from build123d import *

# Parameters (mm, degrees)
SKETCH_1_W          = 140
SKETCH_1_H          = 50
EXTRUDE_1_DEPTH     = 6
SKETCH_6_R          = 2.75
CUT_EXTRUDE_4_DEPTH = 7
SKETCH_5_W          = 140
SKETCH_5_H          = 12
EXTRUDE_3_DEPTH     = 2
M6X1_01_AT_2_COUNT  = 2
M6X1_01_AT_2_PITCH  = 50
M6X1_01_AT_3_COUNT  = 2
M6X1_01_AT_3_PITCH  = 50
SKETCH_4_W          = 9
SKETCH_4_H          = 26
CUT_EXTRUDE_2_DEPTH = 9


with BuildPart() as part:
    # Эскиз1 → Вытянуть1 (new body)
    with BuildSketch(Plane.XY):
        Rectangle(SKETCH_1_W, SKETCH_1_H)
    extrude(amount=EXTRUDE_1_DEPTH)

    # Эскиз6 → Вытянуть4 (cut, through all)
    with BuildSketch(Plane(origin=(0, 0, 0), x_dir=(-1, 0, 0), z_dir=(0, 0, -1))):
        with Locations((42, 19)):
            Circle(SKETCH_6_R)
        with Locations((14, 19)):
            Circle(SKETCH_6_R)
        with Locations((-14, 19)):
            Circle(SKETCH_6_R)
        with Locations((-42, 19)):
            Circle(SKETCH_6_R)
    extrude(amount=-CUT_EXTRUDE_4_DEPTH, mode=Mode.SUBTRACT)

    # Эскиз5 → Вытянуть3 (add)
    with BuildSketch(Plane(origin=(0, 0, 0), x_dir=(-1, 0, 0), z_dir=(0, 0, -1))):
        with Locations((0, -19)):
            Rectangle(SKETCH_5_W, SKETCH_5_H)
    extrude(amount=EXTRUDE_3_DEPTH)

    # Эскиз2 → Отверстие обработанное метчиком M6x1.01 (revolve, cut)
    with BuildSketch(Plane(origin=(0, -19, 6), x_dir=(0, -1, 0), z_dir=(1, 0, 0))):
        Polygon((0, 0), (0, 8.000025), (3.25, 8.000025), (2.5, 7.250025), (2.5, 0), align=None)
    m6x1_01 = revolve(axis=Axis((0, -19, 12.35), (0, 0, -1)), mode=Mode.SUBTRACT)

    # Отверстие обработанное метчиком M6x1.01 at 2: Отверстие обработанное метчиком M6x1.01 ×2
    with Locations(*[(-i * M6X1_01_AT_2_PITCH, 0, 0) for i in range(1, M6X1_01_AT_2_COUNT)]):
        add(m6x1_01, mode=Mode.SUBTRACT)

    # Отверстие обработанное метчиком M6x1.01 at 3: Отверстие обработанное метчиком M6x1.01 ×2
    with Locations(*[(i * M6X1_01_AT_3_PITCH, 0, 0) for i in range(1, M6X1_01_AT_3_COUNT)]):
        add(m6x1_01, mode=Mode.SUBTRACT)

    # Эскиз4 → Вытянуть2 (cut, through all)
    with BuildSketch(Plane.XY.offset(6)):
        with Locations((-65.5, 12)):
            Rectangle(SKETCH_4_W, SKETCH_4_H)
        with Locations((65.5, 12)):
            Rectangle(SKETCH_4_W, SKETCH_4_H)
    extrude(amount=-CUT_EXTRUDE_2_DEPTH, mode=Mode.SUBTRACT)


solid = part.part
Source: CAD feature listing. Evaluate the final solid. Frame: model axes, mm. A direction names the side the tool comes from. Coordinates: 2 decimals unless noted, no trailing zeros. Loops run counter-clockwise (first coordinate to the right, second up) from the corner with the lowest first, then second, coordinate; pieces in that order, holes last. Notation, with made-up numbers: (44.5, 49.25) - (80.5, 49.25) arc R23 cw to (80.5, 83.25) - close; hole circle Ø4 at (25, 88). An arc over 180 degrees is marked (long way). Return JSON: item names as keys, results as strings.
Q1. Section B-B, the plane y = 19. Return loops of the section in (x, z).
Results:
{"outline": "(-61, 0) - (-44.75, 0) - (-44.75, 6) - (-61, 6) - close; (-39.25, 0) - (-16.75, 0) - (-16.75, 6) - (-39.25, 6) - close; (-11.25, 0) - (11.25, 0) - (11.25, 6) - (-11.25, 6) - close; (16.75, 0) - (39.25, 0) - (39.25, 6) - (16.75, 6) - close; (44.75, 0) - (61, 0) - (61, 6) - (44.75, 6) - close"}
Q2. Contact query for flat-ended pins moving along their axis: P1, Ø2, axis at y = 8, z = 5, coming from the +X side; P2, Ø8, axis at x = 39, y = 11.5, coming from the -Z side; P3, Ø3, axis at x = 64.5, z = 3, coming from the +Y side. Output: stop coordinate, or through.
Results:
{"P1": "x = 61", "P2": "z = 0", "P3": "y = -1"}
Q3. Access query for faces 5 (the flat face through (-1, 0, 6)), 6 (the flat face through (61, 12, 3)), 7 (the flat face through (-1, 6, 0)). Directions: +Z, -Z, +X, -X, +Y, -Y. A direction counts if a zero-diameter tool reaches every point of the face in a straight line with its end or side. Return the directions, or none.
Results:
{"face 5": "+Z, +X, -X, +Y, -Y", "face 6": "+Z, -Z, +X, +Y", "face 7": "-Z, +X, -X, +Y"}
Q4. Section D-D, the plane x = 25. Return loops of the section in (y, z).
Results:
{"outline": "(-25, -2) - (-13, -2) - (-13, 0) - (25, 0) - (25, 6) - (-25, 6) - close"}
Q5. Section C-C, the plane z = 4.75. Return loops of the section in (x, y), plus the area to 3 significant figures.
Results:
{"outline": "(-70, -25) - (70, -25) - (70, -1) - (61, -1) - (61, 25) - (-61, 25) - (-61, -1) - (-70, -1) - close; hole circle Ø5 at (-50, -19); hole circle Ø5.5 at (-42, 19); hole circle Ø5.5 at (-14, 19); hole circle Ø5 at (0, -19); hole circle Ø5.5 at (14, 19); hole circle Ø5.5 at (42, 19); hole circle Ø5 at (50, -19)", "area": "6,380 mm2"}
Q6. Section A-A, the plane x = -42. Return loops of the section in (y, z), plus the area to 3 significant figures.
Results:
{"outline": "(-25, -2) - (-13, -2) - (-13, 0) - (16.25, 0) - (16.25, 6) - (-25, 6) - close; (21.75, 0) - (25, 0) - (25, 6) - (21.75, 6) - close", "area": "291 mm2"}
Q7. Mould query, pull axis Y, two halves, no side actions, for faces 1 (the flat face through (-66, -1, 3)), 2 (the cylindrical face through (-13.642, 21.727, 2.958)), 3 (the flat face through (70, -13, 2)), 4 (the cylindrical face through (-0.1, -16.5, 2.4)). Classes: released by +Y, released by -Y, zero draft, split by the parting line, or undercut.
Results:
{"face 1": "released by +Y", "face 2": "undercut", "face 3": "zero draft", "face 4": "undercut"}
Q8. Material intervals for line 1 along X through (y, z) = (-19, 2); line 2 along Y through (x, z) = (-50, 2.5); line 3 along Y through (x, z) = (14, 1.2), sorted ascending.
Results:
{"line 1": "-70 to -52.5, -47.5 to -2.5, 2.5 to 47.5, 52.5 to 70", "line 2": "-25 to -21.5, -16.5 to 25", "line 3": "-25 to 16.25, 21.75 to 25"}
